Input: part model. Units: mm. Frame: model coordinates. Face numbers are marked on the shaded views. A direction names the side the tool comes from. Give positions to 0.01 mm unless a question says otherwise; leave off trailing zeros. Write each loop counter-clockwise with the first axis right and the second up, starting at its lowest first coordinate (ties: lowest second). Pieces come first, ordered by that corner, then holes.
```python
from build123d import *

# Parameters (mm, degrees)
SKETCH1_R           = 6
SKETCH1_R_2         = 2
BOSS_EXTRUDE1_DEPTH = 4
CUT_EXTRUDE2_DEPTH  = 5
CIRPATTERN2_COUNT   = 12


with BuildPart() as part:
    # Sketch1 → Boss-Extrude1 (new body)
    with BuildSketch(Plane.XY):
        Circle(SKETCH1_R)
        Circle(SKETCH1_R_2, mode=Mode.SUBTRACT)
    extrude(amount=BOSS_EXTRUDE1_DEPTH)

    # Sketch4 → Cut-Extrude2 (cut, through all)
    with BuildSketch(Plane.XY):
        with BuildLine():
            ThreePointArc((-0.160215471, 3.996790087), (-0.266788325, 4.035374045), (-0.315943185, 4.137502858))
            ThreePointArc((-0.315943185, 4.137502858), (-0.829511973, 5.435929685), (-2.010193861, 6.181352655))
            ThreePointArc((-2.010193861, 6.181352655), (0, 6.5), (2.010193861, 6.181352655))
            ThreePointArc((2.010193861, 6.181352655), (0.829511973, 5.435929685), (0.315943185, 4.137502858))
            ThreePointArc((0.315943185, 4.137502858), (0.266788325, 4.035374045), (0.160215471, 3.996790087))
            ThreePointArc((0.160215471, 3.996790087), (0, 4), (-0.160215471, 3.996790087))
        make_face()
    cut_extrude2 = extrude(amount=CUT_EXTRUDE2_DEPTH, mode=Mode.SUBTRACT)

    # CirPattern2: Cut-Extrude2 ×12 about axis
    cirpattern2_axis = Axis((0, 0, 0), (0, 0, 1))
    for i in range(1, CIRPATTERN2_COUNT):
        add(cut_extrude2.rotate(cirpattern2_axis, i * 360 / CIRPATTERN2_COUNT), mode=Mode.SUBTRACT)


solid = part.part
```
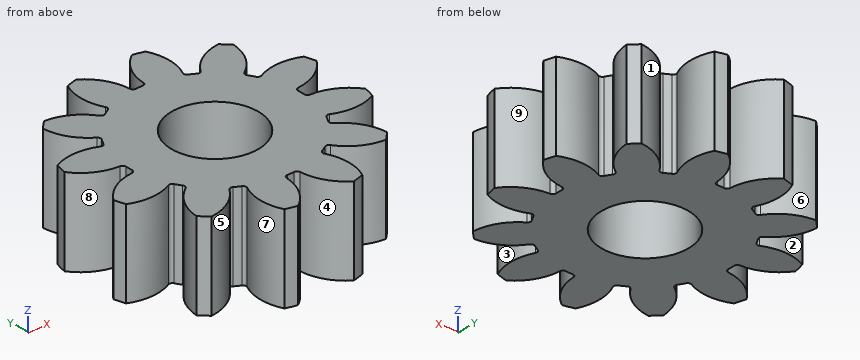
Item 1: Pin query (flat end, axial travel): pin 1 (2.5 mm diameter, centred on x = 0, y = 0, fed in from +Z); pin 2 (1.5 mm diameter, centred on x = -4, z = 0.5, fed in from -Y). Return the tip coordinate at first contact, or that it passes through.
Item 2: Section C-C (y = 2.5). Return loops of the section in (x, z).
Item 3: Mould query, pull axis Y, two halves, no side actions, for the marked faces 1, 2, 3 and 4. Classes: +Y half, -Y half, draft (parallel to the pull), parting line (faces both ways), or undercut.
Item 4: Set-up query: the marked faces 5, 6, 7, 8 and 9. Return all of +Z, -Z, +X, -X, +Y, -Y with unobstructed straight access to the full face (end or side cutting, diameter ignored); none if empty.
Item 5: Ray query, line 1 (Y direction, x = 0, z = 2.2); line 2 (X direction, y = 3.5, z = 2.2); line 3 (X direction, y = -2.25, z = 1.15). Return the intervals inside material, ascending.
Item 6: Section A-A (x = 0). Return loops of the section in (y, z), and give its area (3 significant figures).
Solved:
1. pin 1: passes through
1. pin 2: stops at y = -4.43
2. outline: (-3.64, 0) - (3.64, 0) - (3.64, 4) - (-3.64, 4) - close
3. face 1: +Y half
3. face 2: undercut
3. face 3: undercut
3. face 4: -Y half
4. face 5: +Z, -Z, -Y
4. face 6: +Z, -Z, +Y
4. face 7: +Z, -Z
4. face 8: +Z, -Z, -X
4. face 9: +Z, -Z, +X
5. line 1: y = -4 to -2, 2 to 4
5. line 2: x = -4.32 to -2.39, -1.94 to 1.94, 2.39 to 4.32
5. line 3: x = -3.36 to 3.36
6. outline: (-4, 0) - (-2, 0) - (-2, 4) - (-4, 4) - close; (2, 0) - (4, 0) - (4, 4) - (2, 4) - close
6. area: 16.0 mm2
